Could you check a few things on this model? Use its own coordinates, in mm. Face numbers are marked on the shaded views. A direction names the side the tool comes from. Give positions to 0.01 mm unless a question says otherwise; leave off trailing zeros. Order: outer loops, then holes, each group sorted by start corner. A loop starts at its lowest first (then second) coordinate and runs counter-clockwise, first axis right, second up.
(1) Will these pins go through, and if not, where does the flat tip stop? pin 1 (4 mm diameter, centred on x = -24.5, y = 5.03, fed in from -Z); pin 2 (5 mm diameter, centred on y = 2, z = 32, fed in from -X); pin 3 (19 mm diameter, centred on x = -12.21, z = 39.03, fed in from +Y); pin 4 (7 mm diameter, centred on x = 12.21, z = 39.03, fed in from +Y).
(2) On a 3-axis mill with a long thin cutter (end or side, diameter ignored), from which of +Z, -Z, +X, -X, +Y, -Y can I reach the whole of each face in a straight line? I mean the marked faces 4 and 5. Say none if no direction works.
(3) Imagine slicing it at B-B, the plane z = 24. Write out the boundary of the cut face in (x, y).
(4) Imagine slicing it at D-D, the plane x = -36. Write out the boundary of the cut face in (y, z).
(5) If I drill on probe 1 along X at (y, z) = (7.5, 0); probe 2 along X at (y, z) = (1.5, 40.5); probe 3 along Y at (x, z) = (24.5, 34.75), over which ranges is the centre line in solid material (lowest first)?
(6) If we mould it in two halves opening along X, with no side actions, what happens to the marked faces 1, 2 and 3? For each: released by +X, released by -X, zero draft, split by the parting line, or undercut.
(7) Imagine slicing it at A-A, the plane x = 0. Write out the boundary of the cut face in (y, z).
from build123d import *

# Parameters (mm, degrees)
SKETCH1_R           = 1.75
SKETCH1_R_2         = 6
SKETCH1_R_3         = 1.735302394
BOSS_EXTRUDE1_DEPTH = 10
FILLET2_R           = 3
SKETCH2_R           = 1.3
CUT_EXTRUDE1_DEPTH  = 20


with BuildPart() as part:
    # Sketch1 → Boss-Extrude1 (new body)
    with BuildSketch(Plane(origin=(0, 0, 0), x_dir=(1, 0, 0), z_dir=(0, 1, 0))):
        with BuildLine():
            Line((49.859310292, 3.748223209), (43.664405044, 3.223270017))
            ThreePointArc((43.664405044, 3.223270017), (41.560921763, -13.771692694), (33.099549072, -28.659895126))
            Line((33.099549072, -28.659895126), (-33.099549072, -28.659895126))
            ThreePointArc((-33.099549072, -28.659895126), (-41.560921763, -13.771692694), (-43.664405044, 3.223270017))
            Line((-43.664405044, 3.223270017), (-49.859310292, 3.748223209))
            ThreePointArc((-49.859310292, 3.748223209), (0, -50), (49.859310292, 3.748223209))
        make_face()
        with Locations(Location((-47, 0, 0), (0, 0, 270))):
            Circle(SKETCH1_R, mode=Mode.SUBTRACT)
        with Locations(Location((-12.208117153, -39.030992967, 0), (0, 0, 270))):
            Circle(SKETCH1_R_2, mode=Mode.SUBTRACT)
        with Locations(Location((0, -47, 0), (0, 0, 90))):
            Circle(SKETCH1_R_3, mode=Mode.SUBTRACT)
        with Locations(Location((12.208117153, -39.030992967, 0), (0, 0, 90))):
            Circle(SKETCH1_R_2, mode=Mode.SUBTRACT)
        with Locations(Location((47, 0, 0), (0, 0, 90))):
            Circle(SKETCH1_R, mode=Mode.SUBTRACT)
    extrude(amount=BOSS_EXTRUDE1_DEPTH)

    # Fillet2
    fillet2_edges = [part.edges().sort_by_distance(p)[0] for p in [
        (43.664405044, 5, -3.223270017),
        (49.859310292, 5, -3.748223209),
        (-49.859310292, 5, -3.748223209),
        (-43.664405044, 5, -3.223270017),
    ]]
    fillet(fillet2_edges, radius=FILLET2_R)

    # Sketch2 → Cut-Extrude1 (cut)
    with BuildSketch(Plane(origin=(0, 0, 28.659895126), x_dir=(-1, 0, 0), z_dir=(0, 0, -1))):
        with Locations((24.499993487, 5.025263165)):
            Circle(SKETCH2_R)
        with Locations((-24.5, 5)):
            Circle(SKETCH2_R)
    extrude(amount=-CUT_EXTRUDE1_DEPTH, mode=Mode.SUBTRACT)


solid = part.part
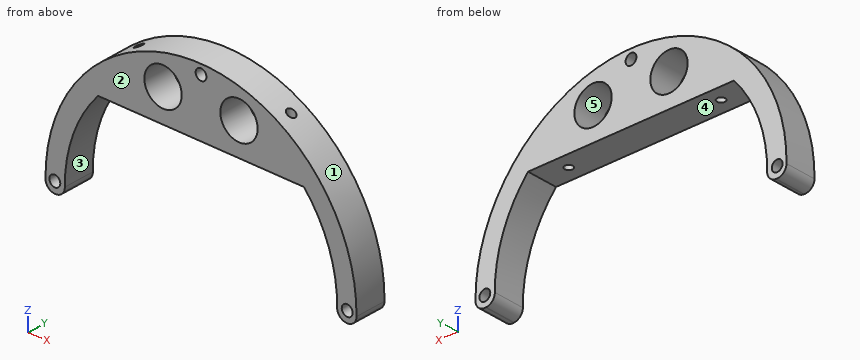
Answer block:
1. pin 1: stops at z = 28.66
1. pin 2: stops at x = -40.37
1. pin 3: stops at y = 10
1. pin 4: passes through
2. face 4: -Z, +Y, -Y
2. face 5: +Y, -Y
3. outline: (-43.86, 0) - (-36.62, 0) - (-36.62, 10) - (-43.86, 10) - close; (36.62, 0) - (43.86, 0) - (43.86, 10) - (36.62, 10) - close
4. outline: (0, 24.92) - (10, 24.92) - (10, 34.7) - (0, 34.7) - close
5. probe 1: x = -50 to -48.75, -45.25 to -43.78, 43.78 to 45.25, 48.75 to 50
5. probe 2: x = -29.32 to -18.03, -6.39 to 6.39, 18.03 to 29.32
5. probe 3: y = 0 to 3.7, 6.3 to 10
6. face 1: split by the parting line
6. face 2: zero draft
6. face 3: undercut
7. outline: (0, 28.66) - (10, 28.66) - (10, 45.26) - (0, 45.26) - close; (0, 48.74) - (10, 48.74) - (10, 50) - (0, 50) - close
